Could you check a few things on this model? Use its own coordinates, in mm. A direction names the side the tool comes from. Coordinates: 2 decimals unless noted, no trailing zeros. Loops run counter-clockwise (first coordinate to the right, second up) from the corner with the lowest first, then second, coordinate; pieces in that order, holes last.
from build123d import *

# Parameters (mm, degrees)
SKETCH1_W           = 63.5
SKETCH1_H           = 127
BOSS_EXTRUDE1_DEPTH = 6.35
SKETCH2_W           = 63.430323736
SKETCH2_H           = 76.2
BOSS_EXTRUDE2_DEPTH = 6.35
SKETCH3_W           = 63.5
SKETCH3_H           = 6.35
BOSS_EXTRUDE3_DEPTH = 6.35
SKETCH4_R           = 44.45
SKETCH4_R_2         = 41.91
BOSS_EXTRUDE4_DEPTH = 63.5


with BuildPart() as part:
    # Sketch1 → Boss-Extrude1 (new body)
    with BuildSketch(Plane.XY):
        with Locations((31.75, -63.5)):
            Rectangle(SKETCH1_W, SKETCH1_H)
    extrude(amount=BOSS_EXTRUDE1_DEPTH)



with BuildPart() as body_2:
    # Sketch2 → Boss-Extrude2 (new body)
    with BuildSketch(Plane.XZ.offset(127)):
        with Locations((31.715161868, 38.1)):
            Rectangle(SKETCH2_W, SKETCH2_H)
    extrude(amount=BOSS_EXTRUDE2_DEPTH)


with BuildPart() as part_1:
    add(part.part)

    add(body_2.part)  # Boss-Extrude3 merges body 2
    # Sketch3 → Boss-Extrude3 (add)
    with BuildSketch(Plane.XZ.offset(127)):
        with Locations((31.75, 3.175)):
            Rectangle(SKETCH3_W, SKETCH3_H)
    extrude(amount=BOSS_EXTRUDE3_DEPTH)

    # Sketch4 → Boss-Extrude4 (add)
    with BuildSketch(Plane(origin=(0, -63.5, 0), x_dir=(1, 0, 0), z_dir=(0, 1, 0))):
        with Locations((32.537747745, -44.45)):
            Circle(SKETCH4_R)
        with Locations((32.537747745, -44.45)):
            Circle(SKETCH4_R_2, mode=Mode.SUBTRACT)
    extrude(amount=-BOSS_EXTRUDE4_DEPTH)


solid = part_1.part
(1) For pin 1 (3 mm diameter, centred on x = 37.5, y = -129, fed in from +Z); pin 2 (10 mm diameter, centred on y = -88, z = 75.5, fed in from -X); pin 3 (25 mm diameter, centred on x = 21.5, z = 65.5, fed in from +Y), each with a flat end and sliding along its axis, tell me the tip position at first contact or that it passes through.
Answers:
pin 1: stops at z = 76.2
pin 2: stops at x = -3.48
pin 3: stops at y = -127
(2) Imagine slicing it at D-D, the plane y = -111. Write out the boundary of the cut face in (x, z).
Answers:
outline: (0, 0) - (63.5, 0) - (63.5, 6.35) - (55.43, 6.35) arc R44.45 ccw (long way) to (9.64, 6.35) - (0, 6.35) - close; hole (15.08, 6.35) - (50, 6.35) arc R41.91 ccw (long way) to start
(3) I need wall thicknesses on probe 1 along X at (y, z) = (-101, 44); probe 2 along Z at (x, y) = (54, -56); probe 3 along Y at (x, z) = (59, 74). Which ranges of each line are inside material? Lowest first, please.
Answers:
probe 1: x = -11.91 to -9.37, 74.45 to 76.99
probe 2: z = 0 to 6.35
probe 3: y = -133.35 to -127
(4) We'd pull the mould along Z, two halves only. Please class faces 5 (the face through (31, -66, 0)), 6 (the face through (64, -127, 73)), 7 (the face through (31, -127, 42)): +Z half, -Z half, draft (parallel to the pull), parting line (faces both ways), or undercut.
Answers:
face 5: -Z half
face 6: draft
face 7: undercut
(5) Imagine slicing it at C-C, the plane z = 80. Write out the boundary of the cut face in (x, y).
Answers:
outline: (5.85, -127) - (10.34, -127) - (10.34, -63.5) - (5.85, -63.5) - close; (54.73, -127) - (59.22, -127) - (59.22, -63.5) - (54.73, -63.5) - close
(6) Imagine slicing it at A-A, the plane z = 44.45. Write out the boundary of the cut face in (x, y).
Answers:
outline: (-11.91, -127) - (-9.37, -127) - (-9.37, -63.5) - (-11.91, -63.5) - close; (0, -133.35) - (63.43, -133.35) - (63.43, -127) - (0, -127) - close; (74.45, -127) - (76.99, -127) - (76.99, -63.5) - (74.45, -63.5) - close
(7) Imagine slicing it at B-B, the plane x = 20. Write out the boundary of the cut face in (y, z).
Answers:
outline: (-133.35, 0) - (0, 0) - (0, 6.35) - (-127, 6.35) - (-127, 76.2) - (-133.35, 76.2) - close; (-127, 84.44) - (-63.5, 84.44) - (-63.5, 87.1) - (-127, 87.1) - close
(8) Which directions (+Z, -Z, +X, -X, +Y, -Y) give clear straight access to the entire face, cutting with the end or side of a thin tool? Please do faces 1 (the face through (30.95, -94.81, 86.33)), 2 (the face through (61, -127, 8)), 3 (the face through (63.5, -68, 3)), 4 (the face through (-10, -127, 47)).
Answers:
face 1: +Y
face 2: +X, +Y
face 3: -Z, +X, +Y, -Y
face 4: +Z, -Z, -X, -Y
